Could you check a few things on this drawing? It's one solid part, dimensions in mm from its lowest x, y, z. Give positions to 0.01 mm unless a question says otherwise; leave off trailing zeros. Write each loop counter-clockwise with the first axis right and the second up, starting at its lowest first coordinate (ties: lowest second). Pieces come first, ordered by that corner, then holes. Notation, with made-up numbers: (40.5, 58.25) -> (54.5, 58.25) arc R24 ccw to (54.5, 84.25) -> close; hole circle Ø8 at (16.5, 77). An arc over 180 degrees is marked (long way). Answer as CSV lines item,"result". Start each with the question number.
1. I need wall thicknesses on line 1 (X direction, y = 6.5, z = 19); line 2 (X direction, y = 12, z = 31.5); line 3 (Z direction, x = 11.25, y = 3). Which ranges of each line are inside material? Lowest first, please. Write a range as [from, to].
2. If we section it at C-C on z = 35: Write out the boundary of the cut face in (x, y), plus the area to 3 significant figures.
3. If we section it at A-A on y = 6.35: Write out the boundary of the cut face in (x, z).
4. I'm going to push flat-ended pins straight in: P1, Ø2, axis at y = 2, z = 28.5, coming from the -X side; P2, Ø6, axis at y = 2, z = 20, coming from the +X side. Where does each tip first touch, or does it pass through?
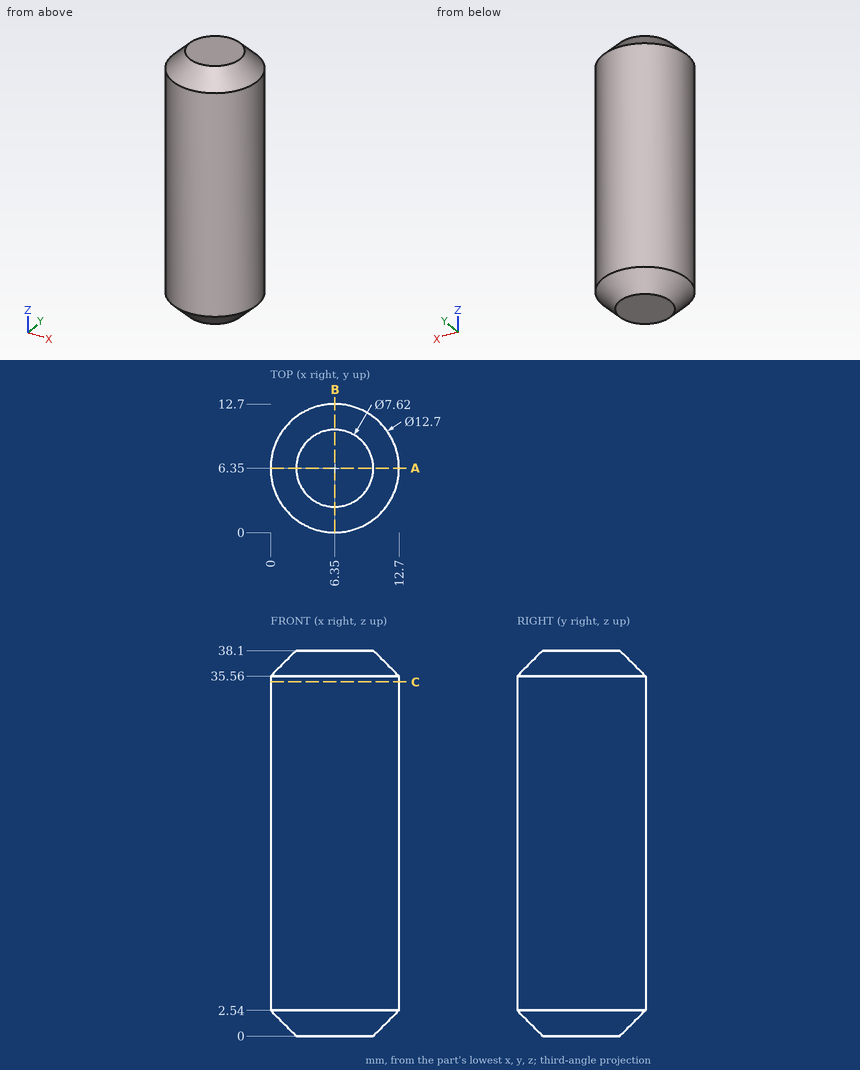
Computed values:
1,line 1,"x = [0, 12.7]"
1,line 2,"x = [3.45, 9.25]"
1,line 3,"z = [2.13, 35.97]"
2,outline,"circle Ø12.7 at (6.35, 6.35)"
2,area,"127 mm2"
3,outline,"(0, 2.54) -> (2.54, 0) -> (10.16, 0) -> (12.7, 2.54) -> (12.7, 35.56) -> (10.16, 38.1) -> (2.54, 38.1) -> (0, 35.56) -> close"
4,P1,"stops at x = 0.96"
4,P2,"stops at x = 12.55"
